```python
from build123d import *

# Parameters (mm, degrees)
BOSS_EXTRUDE1_DEPTH = 25
FILLET1_R           = 1
FILLET2_R           = 1
FILLET3_R           = 0.05
CUT_EXTRUDE1_DEPTH  = 66.934416438
SKETCH5_R           = 7.5
CUT_EXTRUDE2_DEPTH  = 66.193638666


with BuildPart() as part:
    # Sketch2 → Boss-Extrude1 (new body)
    with BuildSketch(Plane.XY):
        with BuildLine():
            Line((-5.6909785, 5.576436412), (-5.6909785, 50))
            Line((-5.6909785, 50), (-6.6909785, 50))
            Line((-6.6909785, 50), (-6.6909785, 4.44447901))
            ThreePointArc((-6.6909785, 4.44447901), (10.790063167, 7.449269771), (28.271104834, 4.44447901))
            Line((28.271104834, 4.44447901), (28.271104834, 49.569009084))
            Line((28.271104834, 49.569009084), (27.271104834, 49.569009084))
            Line((27.271104834, 49.569009084), (27.271104834, 5.576436412))
            ThreePointArc((27.271104834, 5.576436412), (10.790063167, 8.24907617), (-5.6909785, 5.576436412))
        make_face()
    extrude(amount=BOSS_EXTRUDE1_DEPTH)

    # Fillet1
    fillet1_edges = [part.edges().sort_by_distance(p)[0] for p in [
        (-6.6909785, 4.44447901, 12.5),
        (28.271104834, 4.44447901, 12.5),
    ]]
    fillet(fillet1_edges, radius=FILLET1_R)

    # Fillet2
    fillet2_edges = [part.edges().sort_by_distance(p)[0] for p in [
        (-5.6909785, 5.576436412, 12.5),
        (27.271104834, 5.576436412, 12.5),
    ]]
    fillet(fillet2_edges, radius=FILLET2_R)

    # Fillet3
    fillet3_edges = [part.edges().sort_by_distance(p)[0] for p in [
        (-5.6909785, 50, 12.5),
        (-6.6909785, 50, 12.5),
        (28.271104834, 49.569009084, 12.5),
        (27.271104834, 49.569009084, 12.5),
    ]]
    fillet(fillet3_edges, radius=FILLET3_R)

    # Sketch4 → Cut-Extrude1 (cut, through all)
    with BuildSketch(Plane(origin=(28.271104834, 0, 0), x_dir=(0, 0, -1), z_dir=(1, 0, 0))):
        with BuildLine():
            Line((-25, 36.519009084), (-25, 49.519009084))
            Line((-25, 49.519009084), (0, 49.519009084))
            Line((0, 49.519009084), (0, 36.519009084))
            ThreePointArc((0, 36.519009084), (-12.5, 49.019009084), (-25, 36.519009084))
        make_face()
    extrude(amount=-CUT_EXTRUDE1_DEPTH, mode=Mode.SUBTRACT)


with BuildPart() as body_2:
    # of the pieces the cut leaves, the one that is kept (cut_extrude1_keep)
    add(part.part.solids().sort_by_distance((-5.6909785, 6.944623545, 0))[0])

    # Sketch5 → Cut-Extrude2 (cut, through all)
    with BuildSketch(Plane(origin=(28.271104834, 0, 0), x_dir=(0, 0, -1), z_dir=(1, 0, 0))):
        with Locations((-12.5, 36.519009084)):
            Circle(SKETCH5_R)
    extrude(amount=-CUT_EXTRUDE2_DEPTH, mode=Mode.SUBTRACT)


solid = body_2.part
```
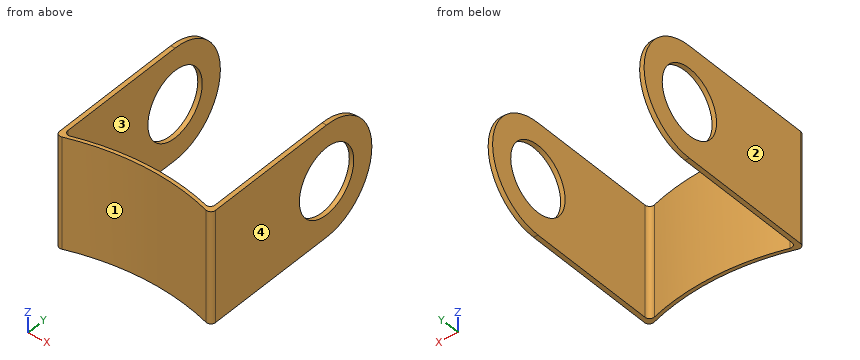
CAD build for the part. Positions are in the model's coordinates, mm. Face numbers are marked on the shaded views. Round coordinates to 2 decimals unless told otherwise and drop trailing zeros. Order: outer loops, then holes, each group sorted by start corner. A loop starts at its lowest first (then second) coordinate and runs counter-clockwise, first axis right, second up. Notation, with made-up numbers: (59.25, -31.5) - (99.25, -31.5) arc R31 cw to (99.25, 5.5) - close; hole circle Ø9 at (7.25, 42.5). An arc over 180 degrees is marked (long way). Use CSV: the item, a comma, the result in double quotes. Start each with the question number.
1) Saw through at D-D (x = 15). List the corners of the cut face in (y, z), and give its area (3 significant figures).
2) Saw through at C-C (z = 9.25). List the corners of the cut face in (x, y), and give its area (3 significant figures).
3) Saw through at B-B (y = 28.5). List the corners of the cut face in (x, z), and give its area (3 significant figures).
4) Pin check, flat tips, straight feed: pin 1 Ø12 at (x, z) = (15, 20) entering from +Y; pin 2 Ø4 at (x, z) = (10.5, 3) entering from -Y; pin 3 Ø2 at (x, z) = (5, 20) entering from -Y. Stop position of each tip, or through.
5) Saw through at A-A (z = 12.5). List the corners of the cut face in (x, y), and give its area (3 significant figures).
6) Wall check: L1, parallel to X at y = 21, z = 23.25; L2, parallel to Y at x = 27.6, z = 12.5; L3, parallel to Y at x = 27.8, z = 12.5. Give the ranges that are in metal, low to high. Write a range as [from, to].
7) Two-plate mould, pull along X, no slides. Class the marked faces 1, 2, 3 and 4: pulls with the +X half, pulls with the -X half, needs draft (parallel to the pull), parting line crosses it, or undercut.
Values follow:
1,outline,"(7.28, 0) - (8.08, 0) - (8.08, 25) - (7.28, 25) - close"
1,area,"20.0 mm2"
2,outline,"(-6.69, 5.84) arc R1 ccw to (-5.38, 4.89) arc R52.35 cw to (26.96, 4.89) arc R1 ccw to (28.27, 5.84) - (28.27, 29.76) - (27.27, 29.76) - (27.27, 6.94) arc R1 cw to (25.98, 5.99) arc R52.15 ccw to (-4.4, 5.99) arc R1 cw to (-5.69, 6.94) - (-5.69, 29.76) - (-6.69, 29.76) - close; (-6.69, 43.28) - (-5.69, 43.28) - (-5.69, 48.59) - (-6.69, 48.59) - close; (27.27, 43.28) - (28.27, 43.28) - (28.27, 48.59) - (27.27, 48.59) - close"
2,area,"87.1 mm2"
3,outline,"(-6.69, 0) - (-5.69, 0) - (-5.69, 25) - (-6.69, 25) - close; (27.27, 0) - (28.27, 0) - (28.27, 25) - (27.27, 25) - close"
3,area,"50.0 mm2"
4,pin 1,"stops at y = 8.25"
4,pin 2,"stops at y = 7.4"
4,pin 3,"stops at y = 7.01"
5,outline,"(-6.69, 5.84) arc R1 ccw to (-5.38, 4.89) arc R52.35 cw to (26.96, 4.89) arc R1 ccw to (28.27, 5.84) - (28.27, 29.02) - (27.27, 29.02) - (27.27, 6.94) arc R1 cw to (25.98, 5.99) arc R52.15 ccw to (-4.4, 5.99) arc R1 cw to (-5.69, 6.94) - (-5.69, 29.02) - (-6.69, 29.02) - close; (-6.69, 44.02) - (-5.69, 44.02) - (-5.69, 49.02) - (-6.69, 49.02) - close; (27.27, 44.02) - (28.27, 44.02) - (28.27, 49.02) - (27.27, 49.02) - close"
5,area,"85.0 mm2"
6,L1,"x = [-6.69, -5.69], [27.27, 28.27]"
6,L2,"y = [4.9, 29.02], [44.02, 49.02]"
6,L3,"y = [4.99, 29.02], [44.02, 49.02]"
7,face 1,"undercut"
7,face 2,"pulls with the -X half"
7,face 3,"undercut"
7,face 4,"pulls with the +X half"
